Autodesk Inventor part; units mm, degrees
ref_plane "Work Plane1" through (5.334, 17.78, 0) normal (1, 0, 0) x (0, 1, 0)
ref_plane "XZ Plane" through (0, 0, 0) normal (0, 1, 0) x (-1, 0, 0)
ref_plane "XY Plane" through (0, 0, 0) normal (0, 0, 1) x (1, 0, 0)
sketch "Sketch2" plane through (0, 0, 0) normal (0, 0, 1) x (1, 0, 0)
  line L0 (0, 0) -> (5.334, 0) construction
  line L1 (5.334, 0) -> (5.334, 35.56) construction
  line L2 (5.334, 35.56) -> (0, 35.56) construction
  line L3 (0, 35.56) -> (0, 0) construction
  line L4 (4.064, 0) -> (4.064, 8.89)
  line L5 (4.064, 8.89) -> (1.7036, 22.2048)
  line L6 (0, 22.86) -> (0.9221, 22.86) construction
  line L7 (0, 8.89) -> (4.064, 8.89) construction
  line L8 (0, 22.86) -> (1.5875, 22.86)
  line L9 (4.064, 0) -> (5.334, 0)
  line L10 (0, 35.56) -> (0, 22.86)
  arc A0 (1.7036, 22.2048) -> (0.9221, 22.86) centre (0.9221, 22.0662) ccw
  line L11 (0, 35.56) -> (5.334, 35.56)
  line L12 (5.334, 35.56) -> (5.334, 0)
  dimension "d6" = 5.334
  dimension "d7" = 4.064
  dimension "d8" = 13.97
  dimension "d9" = 1.5875
  dimension "d10" = 8.89
  dimension "d14" = 0.7937
  dimension "d16" = 12.7
revolve "Revolution2" add sketch "Sketch2" angle 360 about axis through (0, 35.56, 0) along (0, -1, 0)
ref_plane "Work Plane1" through (5.334, 17.78, 0) normal (1, 0, 0) x (0, 1, 0)
sketch "Sketch3" plane through (5.334, 17.78, 0) normal (1, 0, 0) x (0, 1, 0)
  arc A0 (9.3435, 1.5875) -> (9.3435, -1.5875) centre (8.89, 0) ccw
  line L0 (17.78, 5.334) -> (17.78, -5.334) construction
  line L1 (17.78, 0) -> (8.89, 0) construction
  line L2 (17.78, -1.5875) -> (9.3435, -1.5875)
  line L3 (17.78, 1.5875) -> (9.3435, 1.5875)
  line L4 (17.78, 1.5875) -> (17.78, -1.5875)
  point P0 (-17.78, 0)
  dimension "d18" = 3.302
  dimension "d19" = 8.89
  dimension "d21" = 1.5875
extrude "Extrusion1" cut sketch "Sketch3" against normal through all
fillet "Fillet1" radius 3.175 2 edges at (0, 35.56, 1.5875) (0, 35.56, -1.5875)
equation "\"d6\" = shaftRadius + nockWallThickness"
equation "\"d7\" = shaftRadius"
equation "\"d8\" = shaftAngledLength"
equation "\"d9\" = shaftTipRadius"
equation "\"d16\" = knockTotalLength"
equation "\"d18\" = nockStringDiameter"
equation "\"d19\" = nockDepthLengh"
equation "\"d21\" = 0.5 * nockEndWidth"
equation "\"shaftTipDiameter\" = 3.175"
equation "\"shaftDiameter\" = 8.128"
equation "\"shaftAngledLength\" = 13.97"
equation "\"nockTotalLength\" = 31.75"
equation "\"shaftTipRadius\" = 0.5 * shaftTipDiameter"
equation "\"shaftRadius\" = 0.5 * shaftDiameter"
equation "\"nockWallThickness\" = 1.27"
equation "\"knockTotalLength\" = 12.7"
equation "\"nockDepthLengh\" = 8.89"
equation "\"nockStringDiameter\" = 3.302"
equation "\"nockEndWidth\" = 3.175"
properties part number "nockForCalli"
Verification items for the finished model (mm, model axes). A direction names the side the tool comes from. Coordinates: 2 decimals unless noted, no trailing zeros. Order: outer loops, then holes, each group sorted by start corner. A loop starts at its lowest first (then second) coordinate and runs counter-clockwise, first axis right, second up. Notation, with made-up numbers: M 63,88 L 103,88 A14 cw 103,94 Z; hole C 81,73 d4. An arc over 180 degrees is marked long. Return JSON: item names as keys, results as strings.
1) Release check for a two-part mould opening along X. For faces 4 (the flat face through (0, 22.86, 0)), 5 (the cylindrical face through (4.93, 17.53, -2.04)), 6 (the flat face through (0, 30, 1.588)) record: +X half, -X half, draft (parallel to the pull), parting line (faces both ways), or undercut.
Answer list:
{"face 4": "undercut", "face 5": "parting line", "face 6": "draft"}
2) Gauge pin test, flat ends, axial feed: pin 1 (1.5 mm diameter, centred on y = 4.5, z = 3.5, fed in from -X); pin 2 (1 mm diameter, centred on x = 0.5, z = 3.5, fed in from +Y); pin 3 (1.5 mm diameter, centred on x = 0.5, z = 0, fed in from -Y). Record the tip position at first contact, or that the pin passes through.
Answer list:
{"pin 1": "x = -4.57", "pin 2": "y = 35.47", "pin 3": "y = 22.79"}
3) Access from +Z, -Z, +X, -X, +Y, -Y to the whole of each face (thin tool, end or side, straight path). Record for faces 1 (the cylindrical face through (0.07, 25.02, 0.04)), 2 (the cylindrical face through (-0.881, 4.507, 3.967)), 3 (the cylindrical face through (-0.071, 34.605, -2.493)).
Answer list:
{"face 1": "+X, -X", "face 2": "-Y", "face 3": "+X, -X, +Y"}
4) Cross-section at B-B, the plane z = 0. Record the boundary of the cut face in (x, y), and give its area (3 significant figures).
Answer list:
{"outline": "M -5.33,0 L -4.06,0 L -4.06,8.89 L -1.7,22.2 A0.79 cw -0.92,22.86 L 0.92,22.86 A0.79 cw 1.7,22.2 L 4.06,8.89 L 4.06,0 L 5.33,0 L 5.33,25.02 L -5.33,25.02 Z", "area": "116 mm2"}
5) Cross-section at D-D, the plane y = 6.5. Record the boundary of the cut face in (x, z), and give its area (3 significant figures).
Answer list:
{"outline": "C 0,0 d10.67; hole C 0,0 d8.13", "area": "37.5 mm2"}
6) Cross-section at A-A, the plane y = 31. Record the boundary of the cut face in (x, z), and give its area (3 significant figures).
Answer list:
{"outline": "M -5.09,-1.59 A5.33 ccw 5.09,-1.59 Z; M -5.09,1.59 L 5.09,1.59 A5.33 ccw Z", "area": "56.0 mm2"}
7) Thickness scan on L1, parallel to Z at x = 0, y = 28; L2, parallel to Z at x = 0.25, y = 3; L3, parallel to Y at x = 0.5, z = 0. Record the ranges inside material, lowest first. Write a range as [from, to].
Answer list:
{"L1": "[-5.33, -1.59], [1.59, 5.33]", "L2": "[-5.33, -4.06], [4.06, 5.33]", "L3": "[22.86, 25.02]"}
